For this review, take the finished solid that the model builds, in its own axes (mm). Face numbers are marked on the shaded views. A direction names the side the tool comes from. Give positions to 0.01 mm unless a question says otherwise; leave off trailing zeros. Loops run counter-clockwise (first coordinate to the right, second up) from the corner with the lowest first, then second, coordinate; pieces in that order, holes last. Notation, with made-up numbers: (-7, 24.25) -> (43, 24.25) arc R10 cw to (43, 39.25) -> close; hole circle Ø4 at (72.25, 59). An arc over 180 degrees is marked (long way). One line per question, with ' | ' between items. Start each with the question number.
(1) Consider section D-D (y = -4). Write out the cut boundary in (x, z).
(2) Tool access review of the marked faces 5 and 6: name each direction out of +Z, -Z, +X, -X, +Y, -Y from which nothing blocks a thin tool from reaching the whole face with its end or side.
(3) Wall thickness on probe 1 along Y at (x, z) = (-10.5, 68.5); probe 2 along X at (y, z) = (12.5, 49); probe 3 along Y at (x, z) = (-30, 55.5): over which ranges is each line inside the solid? List them lowest first.
(4) Draft analysis for pull direction Y (two halves, no side actions). For the marked faces 1, 2, 3 and 4, state which applies: +Y half, -Y half, draft (parallel to the pull), parting line (faces both ways), or undercut.
(5) Consider section A-A (y = 17.5). Write out the cut boundary in (x, z), and give its area (3 significant figures).
(6) Consider section B-B (z = 37.5). Write out the cut boundary in (x, y), and give its area (3 significant figures).
(7) Insertion check: P1, Ø0.8, axis at x = 13.5, y = -14.5, coming from the -Z side. The pin has a flat end and moves straight along its axis. Give the tip position at first contact, or say it passes through.
(8) Consider section C-C (x = -16). Write out the cut boundary in (y, z), and give its area (3 significant figures).
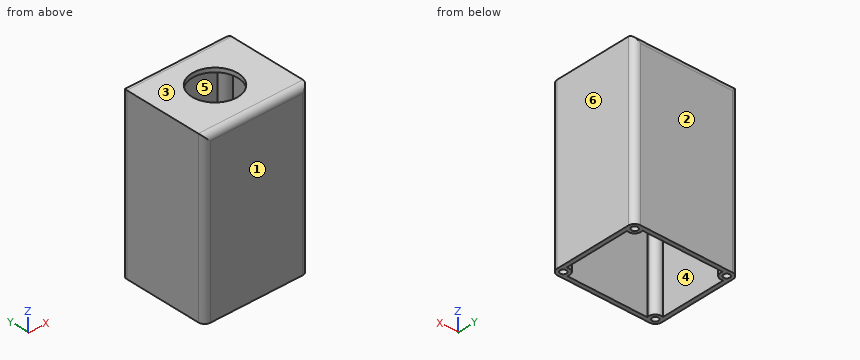
from build123d import *

# Parameters (mm, degrees)
F0_W     = 50
F0_H     = 43
F0_R     = 1.5
F1_DEPTH = 80
F3_T     = -2
F2_R     = 11
F4_DEPTH = 3.1
F5_R     = 3
F6_R     = 1.5
F7_DEPTH = 77
F8_DEPTH = 40


# Not quite as in the source:
# - a feature names something its author has since deleted; it is built from what else it names


with BuildPart() as f1:
    # F0 (on Top) → F1 (new body)
    with BuildSketch(Plane.XY):
        with Locations((-9.0278687937, 4.7237686813)):
            Rectangle(F0_W, F0_H)
        with Locations((-31.0278687937, -13.7762313187)):
            Circle(F0_R, mode=Mode.SUBTRACT)
        with Locations((12.9721312063, -13.7762313187)):
            Circle(F0_R, mode=Mode.SUBTRACT)
        with Locations((-31.0278687937, 23.2237686813)):
            Circle(F0_R, mode=Mode.SUBTRACT)
        with Locations((12.9721312063, 23.2237686813)):
            Circle(F0_R, mode=Mode.SUBTRACT)
        with Locations((12.9721312063, 23.2237686813)):
            Circle(F0_R)
        with Locations((12.9721312063, -13.7762313187)):
            Circle(F0_R)
        with Locations((-31.0278687937, -13.7762313187)):
            Circle(F0_R)
        with Locations((-31.0278687937, 23.2237686813)):
            Circle(F0_R)
    extrude(amount=F1_DEPTH)

    # F3
    f3_openings = [f1.faces().sort_by_distance(p)[0] for p in [
        (-9.027869, 4.723769, 0),
    ]]
    offset(amount=F3_T, openings=f3_openings)

    # F2 (on face) → F4 (cut)
    with BuildSketch(Plane.XY.offset(80)):
        with Locations((-9.0278687937, 4.7237686813)):
            Circle(F2_R)
    extrude(amount=-F4_DEPTH, mode=Mode.SUBTRACT)

    # F5
    f5_edges = [f1.edges().sort_by_distance(p)[0] for p in [
        (15.972131, 26.223769, 40),
        (-9.027869, 26.223769, 80),
        (-34.027869, 26.223769, 40),
        (15.972131, -16.776231, 40),
        (-9.027869, -16.776231, 80),
        (-34.027869, -16.776231, 40),
    ]]
    fillet(f5_edges, radius=F5_R)

    # F6 (on face) → F7 (join)
    with BuildSketch(Plane.XY):
        with BuildLine():
            ThreePointArc((12.9721312104, -16.7762313187), (15.0934515513, -15.8975516608), (15.9721312063, -13.7762313187))
            ThreePointArc((15.9721312063, -13.7762313187), (10.8508108613, -11.6549109766), (12.9721312104, -16.7762313187))
        make_face()
        with Locations((12.9721312063, -13.7762313187)):
            Circle(F6_R, mode=Mode.SUBTRACT)
        with BuildLine():
            ThreePointArc((12.9721312063, 26.2237686813), (10.8508108627, 21.1024483377), (15.9721312063, 23.2237686813))
            ThreePointArc((15.9721312063, 23.2237686813), (15.0934515498, 25.3450890248), (12.9721312063, 26.2237686813))
        make_face()
        with Locations((12.9721312063, 23.2237686813)):
            Circle(F6_R, mode=Mode.SUBTRACT)
        with BuildLine():
            ThreePointArc((-34.0278687937, -13.776231286), (-33.1491891488, -15.8975516507), (-31.0278687937, -16.7762313187))
            ThreePointArc((-31.0278687937, -16.7762313187), (-28.9065484502, -15.8975516623), (-28.0278687937, -13.7762313187))
            ThreePointArc((-28.0278687937, -13.7762313187), (-31.0278687774, -10.7762313187), (-34.0278687937, -13.776231286))
        make_face()
        with Locations((-31.0278687937, -13.7762313187)):
            Circle(F6_R, mode=Mode.SUBTRACT)
        with BuildLine():
            ThreePointArc((-28.0278687937, 23.2237686813), (-28.9065484366, 25.3450890113), (-31.0278687555, 26.2237686813))
            ThreePointArc((-31.0278687555, 26.2237686813), (-33.1491891237, 25.3450890384), (-34.0278687937, 23.2237686813))
            ThreePointArc((-34.0278687937, 23.2237686813), (-31.0278687937, 20.2237686813), (-28.0278687937, 23.2237686813))
        make_face()
        with Locations((-31.0278687937, 23.2237686813)):
            Circle(F6_R, mode=Mode.SUBTRACT)
    extrude(amount=F7_DEPTH)

    # F0 (on Top) → F8 (cut)
    with BuildSketch(Plane.XY):
        with Locations((-31.0278687937, 23.2237686813)):
            Circle(F0_R)
        with Locations((12.9721312063, 23.2237686813)):
            Circle(F0_R)
        with Locations((-31.0278687937, -13.7762313187)):
            Circle(F0_R)
        with Locations((12.9721312063, -13.7762313187)):
            Circle(F0_R)
    extrude(amount=F8_DEPTH, mode=Mode.SUBTRACT)


solid = f1.part
A:
1) outline: (-34.03, 0) -> (-32.03, 0) -> (-32.03, 78) -> (-15.73, 78) -> (-15.73, 80) -> (-34.03, 80) -> close; (-2.33, 78) -> (13.97, 78) -> (13.97, 0) -> (15.97, 0) -> (15.97, 80) -> (-2.33, 80) -> close
2) face 5: -Z | face 6: +Z, -Z, +X, +Y, -Y
3) probe 1: y = -16.78 to -14.78, 24.22 to 26.22 | probe 2: x = -34.03 to -32.03, 13.97 to 15.97 | probe 3: y = -16.78 to -14.78, -12.68 to -10.96, 20.41 to 22.13, 24.22 to 26.22
4) face 1: -Y half | face 2: +Y half | face 3: draft | face 4: undercut
5) outline: (-34.03, 0) -> (-32.03, 0) -> (-32.03, 78) -> (13.97, 78) -> (13.97, 0) -> (15.97, 0) -> (15.97, 80) -> (-34.03, 80) -> close | area: 412 mm^2
6) outline: (-34.03, -13.78) arc R3 ccw to (-31.03, -16.78) -> (12.97, -16.78) arc R3 ccw to (15.97, -13.78) -> (15.97, 23.22) arc R3 ccw to (12.97, 26.22) -> (-31.03, 26.22) arc R3 ccw to (-34.03, 23.22) -> close; hole circle Ø3 at (-31.03, -13.78); hole circle Ø3 at (-31.03, 23.22); hole (-32.03, -10.95) arc R3 cw to (-28.2, -14.78) -> (10.14, -14.78) arc R3 cw to (13.97, -10.95) -> (13.97, 20.4) arc R3 cw to (10.14, 24.22) -> (-28.2, 24.22) arc R3 cw to (-32.03, 20.4) -> close; hole circle Ø3 at (12.97, -13.78); hole circle Ø3 at (12.97, 23.22) | area: 376 mm^2
7) P1: stops at z = 40
8) outline: (-16.78, 0) -> (-14.78, 0) -> (-14.78, 78) -> (-3.78, 78) -> (-3.78, 80) -> (-13.78, 80) arc R3 ccw to (-16.78, 77) -> close; (13.23, 78) -> (24.22, 78) -> (24.22, 0) -> (26.22, 0) -> (26.22, 77) arc R3 ccw to (23.22, 80) -> (13.23, 80) -> close | area: 360 mm^2
